CAD build for the part. Positions are in the model's coordinates, mm. A direction names the side the tool comes from. Coordinates: 2 decimals unless noted, no trailing zeros. Loops run counter-clockwise (first coordinate to the right, second up) from the corner with the lowest first, then second, coordinate; pieces in that order, holes last.
1) Which spindle directions (+Z, -Z, +X, -X, +Y, -Y) get a long thin tool onto all of the face, cutting with end or side? Do faces 4 (the flat face through (-9, -2, 38)), 5 (the flat face through (-12.5, -1, -1)), 6 (the flat face through (8.358, -2, 39)), 7 (the flat face through (0, 0, -37)). Say none if no direction does.
2) Saw through at C-C, the plane y = -29. Write the cut outline in (x, z).
3) Saw through at A-A, the plane x = 6.25. Write the cut outline in (y, z).
4) Two-plate mould, pull along Z, no slides. Class faces 1 (the flat face through (0, 37.5, 1)), 2 (the flat face through (10.383, -2, 0)), 3 (the flat face through (0, -1, -40)): +Z half, -Z half, draft (parallel to the pull), parting line (faces both ways), or undercut.
5) Pin check, flat tip, straight feed: pin 1 Ø1.5 at (x, y) = (-1.5, -36) entering from +Z. Stop position of the tip, or through.
6) Wall check: line 1 along Y through (x, z) = (-6, -31.5); line 2 along X through (y, z) = (-19, -29); line 3 along Z through (x, y) = (-9.75, -5). Give the ranges that are in metal, low to high.
7) Saw through at B-B, the plane z = 29. Write the cut outline in (x, y).
```python
from build123d import *

# Parameters (mm, degrees)
F0_W     = 25
F0_H     = 80
F1_DEPTH = 37.5
F3_DEPTH = 72
F4_W     = 20.765108
F4_H     = 69
F5_DEPTH = 73


with BuildPart() as f1:
    # F0 (on Front) → F1 (new body, symmetric)
    with BuildSketch(Plane.XZ):
        Rectangle(F0_W, F0_H)
    extrude(amount=F1_DEPTH, both=True)

    # F2 (on face) → F3 (cut)
    with BuildSketch(Plane.XZ.offset(37.5)):
        Polygon((8.357823, 38), (8.357823, 40), (0, 40), (-8.357823, 40), (-8.357823, 38), (-10.382554, 38), (-10.382554, 36), (0, 36), (10.382554, 36), (10.382554, 38), align=None)
    extrude(amount=-F3_DEPTH, mode=Mode.SUBTRACT)

    # F4 (on face) → F5 (cut)
    with BuildSketch(Plane.XY.offset(36)):
        Rectangle(F4_W, F4_H)
    extrude(amount=-F5_DEPTH, mode=Mode.SUBTRACT)


solid = f1.part
```
Data:
1. face 4: -Y
1. face 5: +Z, -Z, -X, +Y, -Y
1. face 6: +Z, -Y
1. face 7: none
2. outline: (-12.5, -40) - (12.5, -40) - (12.5, 40) - (8.36, 40) - (8.36, 38) - (10.38, 38) - (10.38, -37) - (-10.38, -37) - (-10.38, 38) - (-8.36, 38) - (-8.36, 40) - (-12.5, 40) - close
3. outline: (-37.5, -40) - (37.5, -40) - (37.5, 40) - (34.5, 40) - (34.5, -37) - (-34.5, -37) - (-34.5, 36) - (-37.5, 36) - close
4. face 1: draft
4. face 2: undercut
4. face 3: -Z half
5. pin 1: stops at z = 36
6. line 1: y = -37.5 to -34.5, 34.5 to 37.5
6. line 2: x = -12.5 to -10.38, 10.38 to 12.5
6. line 3: z = -40 to -37, 38 to 40
7. outline: (-12.5, -37.5) - (12.5, -37.5) - (12.5, 37.5) - (-12.5, 37.5) - close; hole (-10.38, -34.5) - (10.38, -34.5) - (10.38, 34.5) - (-10.38, 34.5) - close
